Read the model definition and answer for the solid it produces. Units are mm, in the model's axes. Face numbers are marked on the shaded views. A direction names the side the tool comes from. Give positions to 0.01 mm unless a question says otherwise; leave off trailing zeros. Loops run counter-clockwise (first coordinate to the right, second up) from the corner with the lowest first, then second, coordinate; pieces in that order, holes last. Notation, with made-up numbers: (74.5, -7.75) - (108.5, -7.75) arc R20 ccw to (108.5, 5.25) - close; hole circle Ø5 at (59, 83). An arc over 180 degrees is marked (long way). Use a Markdown table: item, result. Add a question column.
Item 1: Each of these flat-tipped pins is pushed along its axis until it touches: P1, Ø2.5, axis at x = 15, z = -5, coming from the -Y side; P2, Ø10, axis at y = -20, z = -12, coming from the -X side; P3, Ø17.5, axis at x = 4, z = 1, coming from the -Y side; P4, Ø8, axis at y = -10, z = -8, coming from the +X side. Where does it stop, or does it pass through?
Item 2: A cutting plane is placed at D-D (x = 7). Determine the outline of the cut face in (y, z).
Item 3: For a pull along Z with two mould halves and no side action, classify the marked faces 3, 4, 5 and 6 as +Z half, -Z half, draft (parallel to the pull), parting line (faces both ways), or undercut.
Item 4: A cutting plane is placed at B-B (y = -11.5). Determine the outline of the cut face in (x, z).
Item 5: Consider probe 1 along X at (y, z) = (-1.9, 5); probe 2 along Z at (x, y) = (2.5, -13); probe 3 along Y at (x, z) = (0, -13.2). Determine where each line is inside the solid, lowest interval first. Write a range as [from, to].
Item 6: A cutting plane is placed at C-C (x = 15.5). Determine the outline of the cut face in (y, z).
Item 7: Which of the six approach directions +Z, -Z, +X, -X, +Y, -Y give full straight-line access (tool end or side, diameter ignored) to the marked faces 1 and 2?
Item 8: A cutting plane is placed at A-A (z = 5). Determine the outline of the cut face in (x, y), plus the area to 3 significant figures.
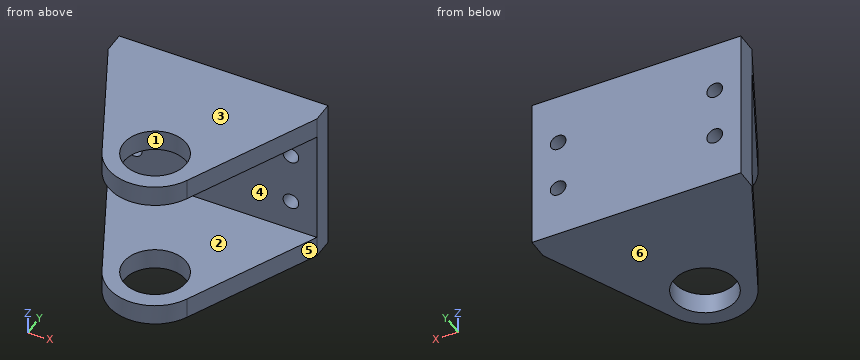
from build123d import *

# Parameters (mm, degrees)
SKETCH_1_W          = 40
SKETCH_1_H          = 20
EXTRUDE_1_DEPTH     = 4
SKETCH_2_R          = 6
EXTRUDE_2_DEPTH     = 5
SKETCH_3_W          = 40
SKETCH_3_H          = 35
CUT_EXTRUDE_1_DEPTH = 1
SKETCH_6_R          = 1.5
CUT_EXTRUDE_3_DEPTH = 10


with BuildPart() as part:
    # 草图1 → 凸台-拉伸1 (new body)
    with BuildSketch(Plane(origin=(0, 0, 0), x_dir=(1, 0, 0), z_dir=(0, 1, 0))):
        Rectangle(SKETCH_1_W, SKETCH_1_H)
    extrude(amount=-EXTRUDE_1_DEPTH)

    # 草图2 → 凸台-拉伸2 (add)
    with BuildSketch(Plane.XY.offset(10)):
        with BuildLine():
            Line((20, -4), (20, 0))
            Line((20, 0), (-20, 0))
            Line((-20, 0), (-20, -4))
            Line((-20, -4), (-8.121724647, -28.877832997))
            ThreePointArc((-8.121724647, -28.877832997), (0, -34), (8.121724647, -28.877832997))
            Line((8.121724647, -28.877832997), (20, -4))
        make_face()
        with Locations((0, -25)):
            Circle(SKETCH_2_R, mode=Mode.SUBTRACT)
    extrude_2 = extrude(amount=EXTRUDE_2_DEPTH)

    # 草图3 → 切除-拉伸1 (cut)
    with BuildSketch(Plane(origin=(0, 0, 10), x_dir=(-1, 0, 0), z_dir=(0, 0, -1))):
        with Locations((0, -21.5)):
            Rectangle(SKETCH_3_W, SKETCH_3_H)
    cut_extrude_1 = extrude(amount=-CUT_EXTRUDE_1_DEPTH, mode=Mode.SUBTRACT)

    # 镜向1: 凸台-拉伸2, 切除-拉伸1 across plane
    add(extrude_2.mirror(Plane.XY))
    add(cut_extrude_1.mirror(Plane.XY), mode=Mode.SUBTRACT)

    # 草图6 → 切除-拉伸3 (cut)
    with BuildSketch(Plane.XZ.offset(4)):
        with Locations(Location((-15, 5, 0), (0, 0, 270))):
            Circle(SKETCH_6_R)
        with Locations(Location((15, 5, 0), (0, 0, 270))):
            Circle(SKETCH_6_R)
        with Locations(Location((-15, -5, 0), (0, 0, 270))):
            Circle(SKETCH_6_R)
        with Locations(Location((15, -5, 0), (0, 0, 270))):
            Circle(SKETCH_6_R)
    extrude(amount=-CUT_EXTRUDE_3_DEPTH, mode=Mode.SUBTRACT)


solid = part.part
Geometry says:
| question | item | result |
|---|---|---|
| 1 | P1 | through |
| 1 | P2 | x = -14.75 |
| 1 | P3 | y = -4 |
| 1 | P4 | x = 18.4 |
| 2 | outline | (-30.66, -15) - (0, -15) - (0, 15) - (-30.66, 15) - (-30.66, 11) - (-4, 11) - (-4, -11) - (-30.66, -11) - close |
| 3 | face 3 | +Z half |
| 3 | face 4 | undercut |
| 3 | face 5 | draft |
| 3 | face 6 | -Z half |
| 4 | outline | (-16.42, -15) - (16.42, -15) - (16.42, -11) - (-16.42, -11) - close; (-16.42, 11) - (16.42, 11) - (16.42, 15) - (-16.42, 15) - close |
| 5 | probe 1 | [-20, -16.5], [-13.5, 13.5], [16.5, 20] |
| 5 | probe 2 | [-15, -11], [11, 15] |
| 5 | probe 3 | [-34, -31], [-19, 0] |
| 6 | outline | (-13.42, -15) - (0, -15) - (0, -6.41) - (-4, -6.41) - (-4, -11) - (-13.42, -11) - close; (-13.42, 11) - (-4, 11) - (-4, 6.41) - (0, 6.41) - (0, 15) - (-13.42, 15) - close; (-4, -3.59) - (0, -3.59) - (0, 3.59) - (-4, 3.59) - close |
| 7 | face 1 | +Z, -Z |
| 7 | face 2 | +X, -X, -Y |
| 8 | outline | (-20, -4) - (-16.5, -4) - (-16.5, 0) - (-20, 0) - close; (-13.5, -4) - (13.5, -4) - (13.5, 0) - (-13.5, 0) - close; (16.5, -4) - (20, -4) - (20, 0) - (16.5, 0) - close |
| 8 | area | 136 mm² |
